from build123d import *

# Parameters (mm, degrees)
SKETCH1_R               = 12.25
SKETCH1_R_2             = 10.5
BOSS_EXTRUDE1_DEPTH     = 62
SKETCH2_R               = 12.25
BOSS_EXTRUDE2_DEPTH     = 3
SKETCH8_W               = 14
SKETCH8_H               = 14
SKETCH8_R               = 0.5
BOSS_EXTRUDE5_DEPTH     = 2.5
SKETCH9_W               = 7
SKETCH9_H               = 7
CUT_EXTRUDE3_DEPTH      = 1
CUT_EXTRUDE3_DEPTH_BACK = 68.5


with BuildPart() as part:
    # Sketch1 → Boss-Extrude1 (new body)
    with BuildSketch(Plane(origin=(0, 0, 0), x_dir=(1, 0, 0), z_dir=(0, 1, 0))):
        Circle(SKETCH1_R)
        Circle(SKETCH1_R_2, mode=Mode.SUBTRACT)
    extrude(amount=BOSS_EXTRUDE1_DEPTH)

    # Sketch2 → Boss-Extrude2 (add)
    with BuildSketch(Plane(origin=(0, 62, 0), x_dir=(1, 0, 0), z_dir=(0, 1, 0))):
        Circle(SKETCH2_R)
    extrude(amount=BOSS_EXTRUDE2_DEPTH)

    # Sketch8 → Boss-Extrude5 (add)
    with BuildSketch(Plane(origin=(0, 65, 0), x_dir=(1, 0, 0), z_dir=(0, 1, 0))):
        Rectangle(SKETCH8_W, SKETCH8_H)
        with BuildLine():
            Line((-8.5, 3.5), (8.5, 3.5))
            ThreePointArc((8.5, 3.5), (12, 0), (8.5, -3.5))
            Line((8.5, -3.5), (-8.5, -3.5))
            ThreePointArc((-8.5, -3.5), (-12, 0), (-8.5, 3.5))
        make_face()
        with Locations((8.5, 0)):
            Circle(SKETCH8_R, mode=Mode.SUBTRACT)
        with Locations((-8.5, 0)):
            Circle(SKETCH8_R, mode=Mode.SUBTRACT)
    extrude(amount=BOSS_EXTRUDE5_DEPTH)

    # Sketch9 → Cut-Extrude3 (cut, two sides)
    with BuildSketch(Plane(origin=(0, 67.5, 0), x_dir=(1, 0, 0), z_dir=(0, 1, 0))) as cut_extrude3_sk:
        Rectangle(SKETCH9_W, SKETCH9_H)
    extrude(amount=CUT_EXTRUDE3_DEPTH, mode=Mode.SUBTRACT)
    extrude(cut_extrude3_sk.sketch, amount=-CUT_EXTRUDE3_DEPTH_BACK, mode=Mode.SUBTRACT)


solid = part.part
Design review of the part built by this model. Coordinates are the model's own, in mm. A direction names the side the tool comes from. Coordinates: 2 decimals unless noted, no trailing zeros. Order: outer loops, then holes, each group sorted by start corner. A loop starts at its lowest first (then second) coordinate and runs counter-clockwise, first axis right, second up.
Item 1: For faces 1 (the flat face through (0, 66, -7)), 2 (the flat face through (7, 66, -5)), 3 (the flat face through (7, 66, 5)), 4 (the flat face through (0, 66, 7)), 5 (the flat face through (5, 62, 0)), list the 3-axis set-ups (+Z, -Z, +X, -X, +Y, -Y) from which the entire face can be reached by the end or side of a thin tool; tool diameter is ignored.
Item 2: For line 1 (X direction, y = 66.55, z = 0); line 2 (X direction, y = 30.5, z = 0); line 3 (Z direction, x = -0.5, y = 52), list the stretches that pass through material, from the lowest coordinate up.
Item 3: Take a section at A-A, the plane x = 0. Write out the cut boundary in (y, z).
Item 4: For pin 1 Ø0.8 at (x, y) = (-7.5, 66) entering from +Z; pin 2 Ø8 at (y, z) = (14.5, 9) entering from -X; pin 3 Ø1.2 at (x, y) = (-7.5, 66) entering from -Z, all flat-tipped, find the tip position at first contact; note any pin that passes through.
Item 5: Take a section at B-B, the plane y = 33. Write out the cut boundary in (x, z).
Item 6: Take a section at C-C, the plane z = -1.5. Write out the cut boundary in (x, y).
Item 7: Take a section at D-D, the plane z = -6.25. Write out the cut boundary in (x, y), then the cut area to 3 significant figures.
Item 8: The part is to be moulded in two halves that separate along Z. For faces 6 (the flat face through (-8, 66, 3.5)), 7 (the flat face through (3.5, 65, 0)), 8 (the flat face through (0, 65, 3.5)), 9 (the flat face through (-8, 66, -3.5)), say which applies: pulls with the +Z half, pulls with the -Z half, needs draft (parallel to the pull), parting line crosses it, or undercut.
The answers:
1. face 1: -Z, +X, -X, +Y
1. face 2: -Z, +X, +Y
1. face 3: +Z, +X, +Y
1. face 4: +Z, +X, -X, +Y
1. face 5: -Y
2. line 1: x = -12 to -9, -8 to -3.5, 3.5 to 8, 9 to 12
2. line 2: x = -12.25 to -10.5, 10.5 to 12.25
2. line 3: z = -12.24 to -10.49, 10.49 to 12.24
3. outline: (0, -12.25) - (65, -12.25) - (65, -7) - (67.5, -7) - (67.5, -3.5) - (62, -3.5) - (62, -10.5) - (0, -10.5) - close; (0, 10.5) - (62, 10.5) - (62, 3.5) - (67.5, 3.5) - (67.5, 7) - (65, 7) - (65, 12.25) - (0, 12.25) - close
4. pin 1: stops at z = 3.5
4. pin 2: stops at x = -11.18
4. pin 3: stops at z = -7
5. outline: circle Ø24.5 at (0, 0); hole circle Ø21 at (0, 0)
6. outline: (-12.16, 0) - (-10.39, 0) - (-10.39, 62) - (-3.5, 62) - (-3.5, 67.5) - (-11.66, 67.5) - (-11.66, 65) - (-12.16, 65) - close; (3.5, 62) - (10.39, 62) - (10.39, 0) - (12.16, 0) - (12.16, 65) - (11.66, 65) - (11.66, 67.5) - (3.5, 67.5) - close
7. outline: (-10.54, 0) - (-8.44, 0) - (-8.44, 62) - (8.44, 62) - (8.44, 0) - (10.54, 0) - (10.54, 65) - (7, 65) - (7, 67.5) - (-7, 67.5) - (-7, 65) - (-10.54, 65) - close
7. area: 358 mm2
8. face 6: pulls with the +Z half
8. face 7: undercut
8. face 8: undercut
8. face 9: pulls with the -Z half
